Check sheet for the modelled part. Datum: model origin and axes. Units: mm. A direction names the side the tool comes from. Coordinates: 2 decimals unless noted, no trailing zeros. Use one line per item in the form item = value. Start each with the question number.
1. Cross-section at A-A on y = -10. Give the number of separate pieces and of enclosed holes in the cut face, then the cut area to 3 significant figures.
2. Tool access check on faces 1 (the face through (0, 9, 2)), 2 (the face through (14.15, 7.04, 3)). Record the directions out of +Z, -Z, +X, -X, +Y, -Y that give a thin tool (end or side, any length) a straight path to the whole face; none if there is none.
3. Draft check along Y on faces 3 (the face through (14.15, 7.04, 1)), 4 (the face through (-3.47, 15.62, 0.49)), 5 (the face through (0, 0.95, 2)). Enter one of: +Y half, -Y half, draft (parallel to the pull), parting line (faces both ways), or undercut.
4. Go/stop test with flat-tipped pins: pin 1 Ø2 at (x, z) = (10.5, 1) entering from -Y; pin 2 Ø1.5 at (x, z) = (3, 0.5) entering from +Y; pin 3 Ø1 at (x, y) = (6.5, 8.5) entering from +Z; pin 4 Ø1.2 at (x, z) = (9.5, 2) entering from -Y. Record where each tip stops, or that it passes through.
5. Scan lines: line 1 along X through (y, z) = (12, 0.2); line 2 along X through (y, z) = (-11, 2); line 3 along Y through (x, z) = (3, 2.4). Record each from-to range of solid material in increasing order.
Autodesk Inventor part; units mm, degrees
ref_plane "YZ Plane" through (0, 0, 0) normal (1, 0, 0) x (0, 1, 0)
ref_plane "XZ Plane" through (0, 0, 0) normal (0, 1, 0) x (-1, 0, 0)
ref_plane "XY Plane" through (0, 0, 0) normal (0, 0, 1) x (1, 0, 0)
sketch "Sketch1" plane through (0, 0, 0) normal (0, 0, 1) x (1, 0, 0)
  circle A0 centre (0, 0) radius 16
  arc A1 (-1.2247, 0.95) -> (1.2247, 0.95) centre (0, 0) ccw
  line L0 (-1.2247, 0.95) -> (1.2247, 0.95)
  line L1 (-3.5, 0) -> (-14.5, 0)
  line L2 (-3.0311, -1.75) -> (-12.5574, -7.25)
  line L3 (-1.75, -3.0311) -> (-7.25, -12.5574)
  line L4 (0, -3.5) -> (0, -14.5)
  line L5 (1.75, -3.0311) -> (7.25, -12.5574)
  line L6 (3.0311, -1.75) -> (12.5574, -7.25)
  line L7 (3.5, 0) -> (14.5, 0)
  line L8 (3.0311, 1.75) -> (12.5574, 7.25)
  line L9 (1.75, 3.0311) -> (7.25, 12.5574)
  line L10 (0, 3.5) -> (0, 14.5)
  line L11 (-1.75, 3.0311) -> (-7.25, 12.5574)
  line L12 (-3.0311, 1.75) -> (-12.5574, 7.25)
  arc A2 (-3.0311, -1.75) -> (-1.75, -3.0311) centre (0, 0) ccw
  arc A3 (0, -3.5) -> (1.75, -3.0311) centre (0, 0) ccw
  arc A4 (3.0311, -1.75) -> (3.5, 0) centre (0, 0) ccw
  arc A5 (3.0311, 1.75) -> (1.75, 3.0311) centre (0, 0) ccw
  arc A6 (0, 3.5) -> (-1.75, 3.0311) centre (0, 0) ccw
  arc A7 (-3.0311, 1.75) -> (-3.5, 0) centre (0, 0) ccw
  arc A8 (-12.5574, -7.25) -> (-7.25, -12.5574) centre (0, 0) ccw
  arc A9 (0, -14.5) -> (7.25, -12.5574) centre (0, 0) ccw
  arc A10 (12.5574, -7.25) -> (14.5, 0) centre (0, 0) ccw
  arc A11 (12.5574, 7.25) -> (7.25, 12.5574) centre (0, 0) ccw
  arc A12 (0, 14.5) -> (-7.25, 12.5574) centre (0, 0) ccw
  arc A13 (-12.5574, 7.25) -> (-14.5, 0) centre (0, 0) ccw
  dimension "d0" = 32
  dimension "d1" = 3.1
  dimension "d2" = 0.95
  dimension "d18" = 360
  dimension "d20" = 14.5
extrude "Extrusion1" add sketch "Sketch1" along normal blind 4
ref_plane "Work Plane3" through (-1.2247, 0, 0) normal (0, -1, 0) x (1, 0, 0)
sketch "Sketch4" plane through (-1.2247, 0, 0) normal (0, -1, 0) x (1, 0, 0)
  line L0 (17.2247, 4) -> (-14.7753, 4)
  line L1 (-14.7753, 0) -> (17.2247, 0)
  line L2 (17.2247, 4) -> (-14.7753, 4) construction
  line L3 (1.2247, 4) -> (1.2247, 0) construction
  line L4 (16.2247, 3) -> (17.2247, 3)
  line L5 (17.2247, 3) -> (17.2247, 1)
  line L6 (17.2247, 1) -> (16.2247, 1)
  line L7 (16.2247, 1) -> (16.2247, 3)
  line L8 (17.2247, 0) -> (17.2247, 4)
  line L9 (16.2247, 1) -> (16.2247, 0) construction
  line L10 (16.2247, 3) -> (16.2247, 4) construction
  dimension "d10" = 1
  dimension "d11" = 1
revolve "Revolution1" cut sketch "Sketch4" angle 360 about axis through (0, 0, 4) along (0, 0, -1)
fillet "Fillet1" radius 0.6 2 edges at (-15, 0, 3) (-15, 0, 1)
properties part number "wheel"
Final values:
q1.separate_pieces = 3
q1.enclosed_holes = 0
q1.area = 53.1 mm²
q2.face_1 = +Z, -Z
q2.face_2 = none
q3.face_3 = draft
q3.face_4 = parting line
q3.face_5 = undercut
q4.pin_1 = -12.87
q4.pin_2 = 15.84
q4.pin_3 = through
q4.pin_4 = -12.07
q5.line_1 = -10.58 to -6.93, 0 to 6.93, 8.14 to 10.58
q5.line_2 = -10.2 to -9.45, -6.35 to 0, 6.35 to 10.2
q5.line_3 = -14.7 to -14.19, -5.2 to 1.8, 5.2 to 14.7
